Work out the finished part from the listing and answer in its coordinate system (mm). Round coordinates to 2 decimals unless told otherwise and drop trailing zeros. Loops run counter-clockwise (first coordinate to the right, second up) from the corner with the lowest first, then second, coordinate; pieces in that order, holes last. Notation, with made-up numbers: (48.25, 26.25) - (96.25, 26.25) arc R24 cw to (96.25, 39.25) - close; hole circle Ø7 at (-18.75, 71). An arc over 180 degrees is marked (long way). Return JSON: item names as keys, results as strings.
from build123d import *

# Parameters (mm, degrees)
SCHIZZO1_W                   = 884
SCHIZZO1_H                   = 686
SCHIZZO1_W_2                 = 804
SCHIZZO1_H_2                 = 606
ESTRUSIONE_ESTRUSIONE1_DEPTH = 2.5
SCHIZZO2_R                   = 3.25
TAGLIO_ESTRUSIONE1_DEPTH     = 560.497989273


with BuildPart() as part:
    # Schizzo1 → Estrusione-Estrusione1 (new, symmetric)
    with BuildSketch(Plane(origin=(0, 0, 0), x_dir=(1, 0, 0), z_dir=(0, 1, 0))):
        Rectangle(SCHIZZO1_W, SCHIZZO1_H)
        Rectangle(SCHIZZO1_W_2, SCHIZZO1_H_2, mode=Mode.SUBTRACT)
    extrude(amount=ESTRUSIONE_ESTRUSIONE1_DEPTH, both=True)

    # Schizzo2 → Taglio-Estrusione1 (cut, through all)
    with BuildSketch(Plane(origin=(0, 2.5, 0), x_dir=(1, 0, 0), z_dir=(0, 1, 0))):
        with Locations(Location((-422, 323, 0), (0, 0, 270))):
            Circle(SCHIZZO2_R)
        with Locations(Location((422, 323, 0), (0, 0, 90))):
            Circle(SCHIZZO2_R)
        with Locations(Location((422, -323, 0), (0, 0, 270))):
            Circle(SCHIZZO2_R)
        with Locations(Location((-422, -323, 0), (0, 0, 90))):
            Circle(SCHIZZO2_R)
        with Locations(Location((-282, 323, 0), (0, 0, 270))):
            Circle(SCHIZZO2_R)
        with Locations(Location((-142, 323, 0), (0, 0, 270))):
            Circle(SCHIZZO2_R)
        with Locations(Location((0, 323, 0), (0, 0, 270))):
            Circle(SCHIZZO2_R)
        with Locations(Location((142, 323, 0), (0, 0, 90))):
            Circle(SCHIZZO2_R)
        with Locations(Location((282, 323, 0), (0, 0, 90))):
            Circle(SCHIZZO2_R)
        with Locations(Location((282, -323, 0), (0, 0, 270))):
            Circle(SCHIZZO2_R)
        with Locations(Location((142, -323, 0), (0, 0, 270))):
            Circle(SCHIZZO2_R)
        with Locations(Location((0, -323, 0), (0, 0, 90))):
            Circle(SCHIZZO2_R)
        with Locations(Location((-142, -323, 0), (0, 0, 90))):
            Circle(SCHIZZO2_R)
        with Locations(Location((-282, -323, 0), (0, 0, 90))):
            Circle(SCHIZZO2_R)
        with Locations(Location((-422, 183, 0), (0, 0, 270))):
            Circle(SCHIZZO2_R)
        with Locations(Location((-422, 43, 0), (0, 0, 270))):
            Circle(SCHIZZO2_R)
        with Locations(Location((-422, -43, 0), (0, 0, 90))):
            Circle(SCHIZZO2_R)
        with Locations(Location((-422, -183, 0), (0, 0, 90))):
            Circle(SCHIZZO2_R)
        with Locations(Location((422, -183, 0), (0, 0, 270))):
            Circle(SCHIZZO2_R)
        with Locations(Location((422, -43, 0), (0, 0, 270))):
            Circle(SCHIZZO2_R)
        with Locations(Location((422, 43, 0), (0, 0, 90))):
            Circle(SCHIZZO2_R)
        with Locations(Location((422, 183, 0), (0, 0, 90))):
            Circle(SCHIZZO2_R)
    extrude(amount=-TAGLIO_ESTRUSIONE1_DEPTH, mode=Mode.SUBTRACT)


solid = part.part
1) Section A-A (z = -210.5) is taken. Give the vertices of the cut face in (x, y), and give its area (3 significant figures).
Verdict:
{"outline": "(-442, -2.5) - (-402, -2.5) - (-402, 2.5) - (-442, 2.5) - close; (402, -2.5) - (442, -2.5) - (442, 2.5) - (402, 2.5) - close", "area": "400 mm2"}
2) Section B-B (x = 212.5) is taken. Give the vertices of the cut face in (y, z), and give its area (3 significant figures).
Verdict:
{"outline": "(-2.5, -343) - (2.5, -343) - (2.5, -303) - (-2.5, -303) - close; (-2.5, 303) - (2.5, 303) - (2.5, 343) - (-2.5, 343) - close", "area": "400 mm2"}
3) Section C-C (y = -0.85) is taken. Count the separate pieces of the cut face and the enclosed holes in it, and give its area (3 significant figures).
Verdict:
{"separate pieces": "1", "enclosed holes": "23", "area": "118,000 mm2"}
4) Find the intervals of material crossed by L1, parallel to X at y = 1.15, z = -183; L2, parallel to Z at x = -142, y = 0.8; L3, parallel to Z at x = 149.5, y = -0.8, in increasing order.
Verdict:
{"L1": "x = -442 to -425.25, -418.75 to -402, 402 to 418.75, 425.25 to 442", "L2": "z = -343 to -326.25, -319.75 to -303, 303 to 319.75, 326.25 to 343", "L3": "z = -343 to -303, 303 to 343"}
